Geometry: final body of the model. Coordinates: model frame, mm. Give positions to 0.01 mm unless a question says otherwise; leave off trailing zeros. Write each loop counter-clockwise with the first axis right and the second up, starting at its lowest first coordinate (ties: lowest second). Pieces come first, ordered by that corner, then holes. Notation, with made-up numbers: (28, 70) -> (32, 70) arc R30 cw to (32, 95) -> close; hole circle Ø10 at (0.5, -5.75). An arc over 180 degrees is marked (long way). Answer as a JSON object with one key per item and string values. Group by question number.
(1) Section query C-C on x = 96. Output: boundary loops of the cut face in (y, z).
(2) Material intervals for probe 1 along Z at (x, y) = (-110.5, 0); probe 2 along X at (y, z) = (19.5, 2.5), sorted ascending.
(3) Section query D-D on y = 44.5. Output: boundary loops of the cut face in (x, z).
(4) Contact query for flat-ended pins moving along their axis: pin 1 Ø3 at (x, z) = (-192, 3) entering from -Y; pin 2 Ø4 at (y, z) = (43.5, 1.5) entering from +X; pin 3 Ø10 at (x, y) = (98.5, 27.5) entering from +Z; pin 4 Ø1 at (y, z) = (39, -1) entering from +X. Output: stop coordinate, or through.
(5) Section query B-B on z = 2.5. Output: boundary loops of the cut face in (x, y).
(6) Section query A-A on y = 0. Output: boundary loops of the cut face in (x, z), plus the area to 3 significant figures.
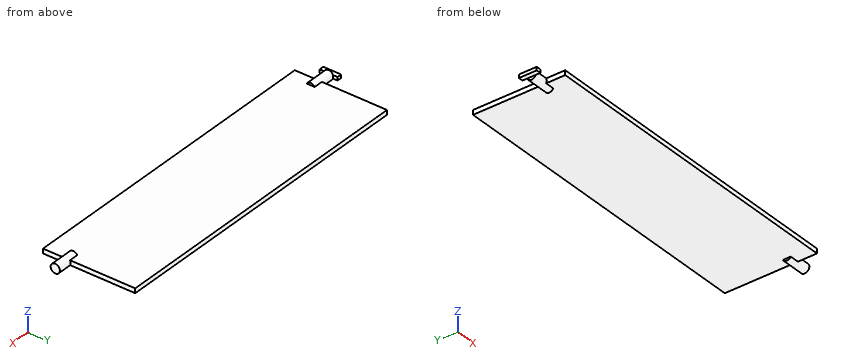
from build123d import *

# Parameters (mm, degrees)
SKETCH1_W           = 350
SKETCH1_H           = 50
BOSS_EXTRUDE1_DEPTH = 5
BOSS_EXTRUDE2_START = -10
SKETCH2_R           = 5
BOSS_EXTRUDE2_DEPTH = 25
SKETCH4_W           = 350
SKETCH4_H           = 5
BOSS_EXTRUDE4_DEPTH = 50
SKETCH5_W           = 3.668837662
SKETCH5_H           = 19.311798598
BOSS_EXTRUDE5_DEPTH = 5


with BuildPart() as part:
    # Sketch1 → Boss-Extrude1 (new body)
    with BuildSketch(Plane.XY):
        Rectangle(SKETCH1_W, SKETCH1_H)
    extrude(amount=BOSS_EXTRUDE1_DEPTH)

    # Sketch2 → Boss-Extrude2 (add)
    with BuildSketch(Plane.ZY.offset(175).offset(BOSS_EXTRUDE2_START)):
        with Locations((2.5, 0)):
            Circle(SKETCH2_R)
    boss_extrude2 = extrude(amount=BOSS_EXTRUDE2_DEPTH)

    # Mirror1: Boss-Extrude2 across plane
    add(boss_extrude2.mirror(Plane(origin=(0, 0, 0), x_dir=(0, 0, 1), z_dir=(1, 0, 0))))

    # Sketch4 → Boss-Extrude4 (add)
    with BuildSketch(Plane(origin=(0, 25, 0), x_dir=(1, 0, 0), z_dir=(0, 1, 0))):
        with Locations((0, -2.5)):
            Rectangle(SKETCH4_W, SKETCH4_H)
    extrude(amount=BOSS_EXTRUDE4_DEPTH)

    # Sketch5 → Boss-Extrude5 (add)
    with BuildSketch(Plane.ZY.offset(190)):
        with Locations((2.5, 0)):
            Rectangle(SKETCH5_W, SKETCH5_H)
    extrude(amount=BOSS_EXTRUDE5_DEPTH)


solid = part.part
Answer list:
{
 "1": {"outline": "(-25, 0) -> (75, 0) -> (75, 5) -> (-25, 5) -> close"},
 "2": {"probe 1": "0 to 5", "probe 2": "-175 to 175"},
 "3": {"outline": "(-175, 0) -> (175, 0) -> (175, 5) -> (-175, 5) -> close"},
 "4": {"pin 1": "y = -9.66", "pin 2": "x = 175", "pin 3": "z = 5", "pin 4": "through"},
 "5": {"outline": "(-195, -9.66) -> (-190, -9.66) -> (-190, -5) -> (-175, -5) -> (-175, -25) -> (175, -25) -> (175, -5) -> (190, -5) -> (190, 5) -> (175, 5) -> (175, 75) -> (-175, 75) -> (-175, 5) -> (-190, 5) -> (-190, 9.66) -> (-195, 9.66) -> close"},
 "6": {"outline": "(-195, 0.67) -> (-190, 0.67) -> (-190, -2.5) -> (-165, -2.5) -> (-165, 0) -> (165, 0) -> (165, -2.5) -> (190, -2.5) -> (190, 7.5) -> (165, 7.5) -> (165, 5) -> (-165, 5) -> (-165, 7.5) -> (-190, 7.5) -> (-190, 4.33) -> (-195, 4.33) -> close", "area": "2,170 mm2"}
}
